from build123d import *

# Parameters (mm, degrees)
SKETCH_1_W          = 364
SKETCH_1_H          = 490
EXTRUDE_1_DEPTH     = 20
SKETCH_2_R          = 13
CUT_EXTRUDE_1_DEPTH = 306.857810101
CHAMFER_1_SIZE      = 10


with BuildPart() as part:
    # 草图1 → 凸台-拉伸1 (new body)
    with BuildSketch(Plane.XY):
        Rectangle(SKETCH_1_W, SKETCH_1_H)
    extrude(amount=EXTRUDE_1_DEPTH)

    # 草图2 → 切除-拉伸1 (cut, through all)
    with BuildSketch(Plane.XY.offset(20)):
        with Locations((-157, 200)):
            Circle(SKETCH_2_R)
        with Locations((-157, 100)):
            Circle(SKETCH_2_R)
        with Locations((-157, 0)):
            Circle(SKETCH_2_R)
        with Locations((-157, -100)):
            Circle(SKETCH_2_R)
        with Locations((-157, -200)):
            Circle(SKETCH_2_R)
        with Locations(Location((157, -200, 0), (0, 0, 180))):
            Circle(SKETCH_2_R)
        with Locations(Location((157, -100, 0), (0, 0, 180))):
            Circle(SKETCH_2_R)
        with Locations(Location((157, 0, 0), (0, 0, 180))):
            Circle(SKETCH_2_R)
        with Locations(Location((157, 100, 0), (0, 0, 180))):
            Circle(SKETCH_2_R)
        with Locations(Location((157, 200, 0), (0, 0, 180))):
            Circle(SKETCH_2_R)
        with BuildLine():
            Line((-71, 175), (71, 175))
            ThreePointArc((71, 175), (78.071067812, 172.071067812), (81, 165))
            Line((81, 165), (81, 45))
            ThreePointArc((81, 45), (78.071067812, 37.928932188), (71, 35))
            Line((71, 35), (-71, 35))
            ThreePointArc((-71, 35), (-78.071067812, 37.928932188), (-81, 45))
            Line((-81, 45), (-81, 165))
            ThreePointArc((-81, 165), (-78.071067812, 172.071067812), (-71, 175))
        make_face()
    extrude(amount=-CUT_EXTRUDE_1_DEPTH, mode=Mode.SUBTRACT)

    # 倒角1
    chamfer_1_edges = [part.edges().sort_by_distance(p)[0] for p in [
        (182, -245, 10),
        (-182, -245, 10),
        (-182, 245, 10),
        (182, 245, 10),
    ]]
    chamfer(chamfer_1_edges, length=CHAMFER_1_SIZE)


solid = part.part
Work out the finished part from the listing and answer in its coordinate system (mm). A direction names the side the tool comes from. Round coordinates to 2 decimals unless told otherwise and drop trailing zeros. Write each loop counter-clockwise with the first axis right and the second up, starting at its lowest first coordinate (ties: lowest second). Pieces come first, ordered by that corner, then holes. Notation, with made-up numbers: (-35, 65.5) -> (5, 65.5) arc R18 cw to (5, 73.5) -> close; hole circle Ø2 at (-14.75, -5.5). An arc over 180 degrees is marked (long way). Write each question's results on one line, items separated by ' | '.
Item 1: Find the intervals of material crossed by line 1 along Y through (x, z) = (-157, 14); line 2 along Y through (x, z) = (-40, 4); line 3 along X through (y, z) = (-10.5, 5), in increasing order. Write a range as [from, to].
Result set:
line 1: [-245, -213], [-187, -113], [-87, -13], [13, 87], [113, 187], [213, 245] | line 2: [-245, 35], [175, 245] | line 3: [-182, -164.66], [-149.34, 149.34], [164.66, 182]
Item 2: The mould has two halves that part along X. Classify faces 3 (the face through (1, 35, 10)), 4 (the face through (182, -3, 10)), 5 (the face through (-145, -105, 10)), 6 (the face through (-3, 3, 20)): +X half, -X half, draft (parallel to the pull), parting line (faces both ways), or undercut.
Result set:
face 3: undercut | face 4: +X half | face 5: undercut | face 6: draft
Item 3: A cutting plane is placed at B-B, the plane x = -157. Determine the outline of the cut face in (y, z).
Result set:
outline: (-245, 0) -> (-213, 0) -> (-213, 20) -> (-245, 20) -> close; (-187, 0) -> (-113, 0) -> (-113, 20) -> (-187, 20) -> close; (-87, 0) -> (-13, 0) -> (-13, 20) -> (-87, 20) -> close; (13, 0) -> (87, 0) -> (87, 20) -> (13, 20) -> close; (113, 0) -> (187, 0) -> (187, 20) -> (113, 20) -> close; (213, 0) -> (245, 0) -> (245, 20) -> (213, 20) -> close
Item 4: Which of the six approach directions +Z, -Z, +X, -X, +Y, -Y give full straight-line access (tool end or side, diameter ignored) to faces 1 (the face through (-81, 104, 10)), 2 (the face through (-177, 240, 10))?
Result set:
face 1: +Z, -Z | face 2: +Z, -Z, -X, +Y
Item 5: A flat-ended cylindrical pin translates along its axis: P1, Ø15.5, axis at x = -157, y = -100, coming from the -Z side. Find the tip coordinate at first contact, or state that the pin passes through.
Result set:
P1: through
Item 6: A cutting plane is placed at D-D, the plane x = -64.5. Determine the outline of the cut face in (y, z), plus the area to 3 significant figures.
Result set:
outline: (-245, 0) -> (35, 0) -> (35, 20) -> (-245, 20) -> close; (175, 0) -> (245, 0) -> (245, 20) -> (175, 20) -> close | area: 7,000 mm^2
Item 7: A cutting plane is placed at C-C, the plane z = 10.25. Count the separate pieces of the cut face and the enclosed holes in it, plus the area to 3 significant figures.
Result set:
separate pieces: 1 | enclosed holes: 11 | area: 150,000 mm^2
Item 8: A cutting plane is placed at A-A, the plane y = -200. Determine the outline of the cut face in (x, z), plus the area to 3 significant figures.
Result set:
outline: (-182, 0) -> (-170, 0) -> (-170, 20) -> (-182, 20) -> close; (-144, 0) -> (144, 0) -> (144, 20) -> (-144, 20) -> close; (170, 0) -> (182, 0) -> (182, 20) -> (170, 20) -> close | area: 6,240 mm^2
